Design review of the part shown in the three views and the two pictorial views. Dimensions are in mm from the part's minimum x, y and z. Give positions to 0.01 mm unless a question says otherwise; leave off trailing zeros. Loops run counter-clockwise (first coordinate to the right, second up) from the corner with the lowest first, then second, coordinate; pieces in that order, holes last. Notation, with made-up numbers: (-29, 27) - (1, 27) arc R21 ccw to (1, 41) - close; hole circle Ø7 at (85, 33). An arc over 180 degrees is marked (long way). Return JSON: item names as keys, results as strings. Group by question number.
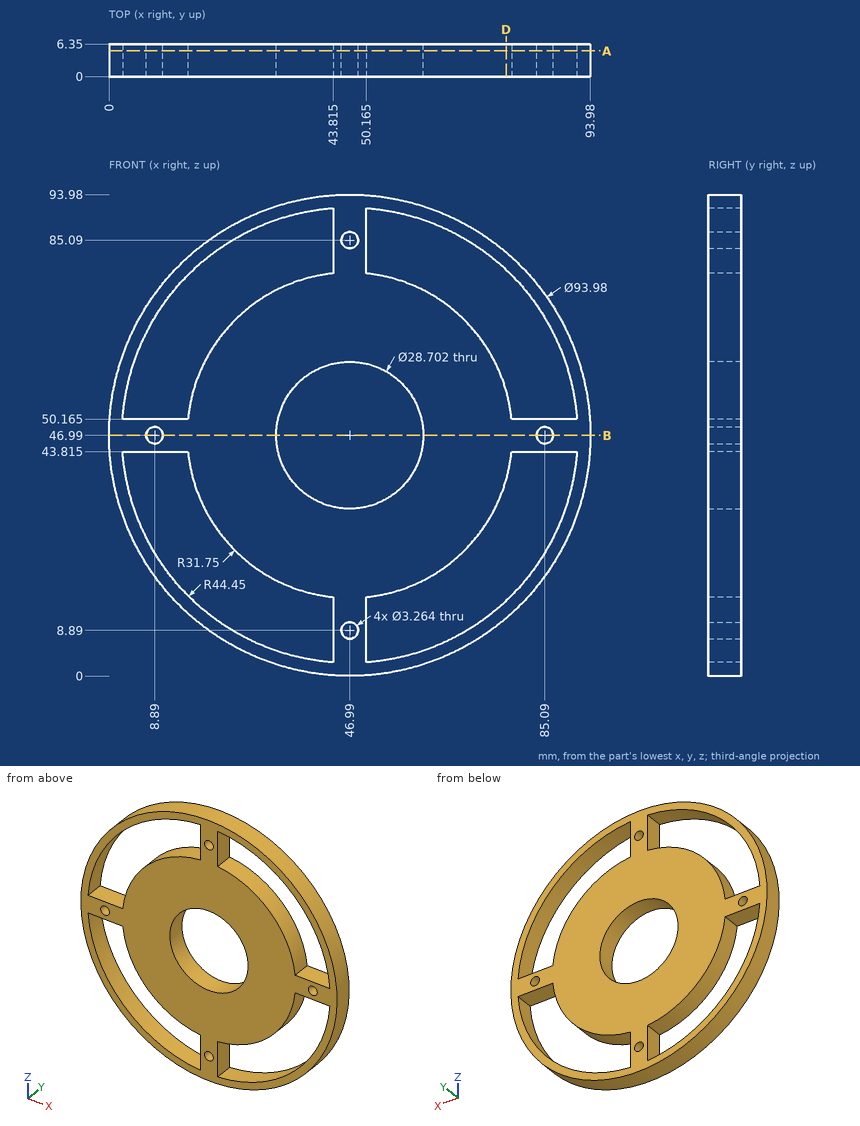
Item 1: Take a section at A-A (y = 5). State how many separate pieces and enclosed holes the cut face has, then the cut area to 3 significant figures.
Item 2: For L1, parallel to X at y = 3.75, z = 40.5; L2, parallel to Z at x = 80.5, y = 2.25 (1 decimal); L3, parallel to Z at x = 9.5, y = 5.25 (1 decimal), list the stretches that pass through material, from the lowest coordinate up. Write a range as from..to.
Item 3: For P1, Ø2, axis at y = 2, z = 40, coming from the -X side; P2, Ø3, axis at y = 3, z = 79, coming from the -X side; P3, Ø2, axis at x = 59.5, y = 5.5, coming from the -Z side, all flat-tipped, find the tip position at first contact; note any pin that passes through.
Item 4: Take a section at D-D (x = 77.5). State the section outline as (y, z) points, then the cut area to 3 significant figures.
Item 5: Take a section at B-B (z = 46.99). State the section outline as (x, y) points.
Check sheet entries:
{
 "1": {"separate pieces": "1", "enclosed holes": "9", "area": "3,540 mm^2"},
 "2": {"L1": "x = 0.45..3.02, 15.91..34.19, 59.79..78.07, 90.96..93.53", "L2": "z = 14..17.8, 43.8..50.2, 76.2..79.9", "L3": "z = 18.7..23.1, 43.8..45.5, 48.5..50.2, 70.9..75.3"},
 "3": {"P1": "stops at x = 0.38", "P2": "stops at x = 11.25", "P3": "stops at z = 1.43"},
 "4": {"outline": "(0, 11.25) - (6.35, 11.25) - (6.35, 14.66) - (0, 14.66) - close; (0, 38.2) - (6.35, 38.2) - (6.35, 55.78) - (0, 55.78) - close; (0, 79.32) - (6.35, 79.32) - (6.35, 82.73) - (0, 82.73) - close", "area": "155 mm^2"},
 "5": {"outline": "(0, 0) - (7.26, 0) - (7.26, 6.35) - (0, 6.35) - close; (10.52, 0) - (32.64, 0) - (32.64, 6.35) - (10.52, 6.35) - close; (61.34, 0) - (83.46, 0) - (83.46, 6.35) - (61.34, 6.35) - close; (86.72, 0) - (93.98, 0) - (93.98, 6.35) - (86.72, 6.35) - close"}
}
